Model file for the job. Use its own axes, mm. Face numbers are marked on the shaded views. A direction names the side the tool comes from. Give positions to 0.01 mm unless a question says otherwise; leave off trailing zeros. Write each loop counter-clockwise with the first axis right and the second up, starting at its lowest first coordinate (ties: lowest second). Pieces come first, ordered by that corner, then holes. Notation, with made-up numbers: (-14, -16) - (19, -16) arc R24 ccw to (19, 0) - close; hole circle Ø10 at (77.25, -16.5). An arc over 180 degrees is marked (long way). One line per item, written item: value. Start each with the question number.
(1) Probe L1, parallel to X at y = 6.5, z = -23; L2, parallel to Z at x = 8, y = 15.5; L3, parallel to X at y = 6.5, z = -20.5. List the from-to ranges inside material, lowest first.
(2) Cut at D-D, the plane x = 8. List the corners of the cut face in (y, z).
(3) Drop flat-ended pins along their axis: P1, Ø9.5, axis at x = 5, y = -4.5, coming from the -Z side; P2, Ø4, axis at x = 25.5, y = 2.5, coming from the +Z side; P3, Ø9.5, axis at y = -5.5, z = -15, coming from the +X side; P4, Ø4, axis at x = 26, z = -18.5, coming from the +Y side. Give the stop position or say it passes through.
(4) 3-axis set-ups, long thin cutter, end or side, ignore diameter. For the marked faces 4, 5 and 6: which of +Z, -Z, +X, -X, +Y, -Y reach the whole face in a straight line?
(5) Cut at C-C, the plane y = -5. List the corners of the cut face in (x, z), and give its area (3 significant figures).
(6) Cut at A-A, the plane y = 2. List the corners of the cut face in (x, z), and give its area (3 significant figures).
(7) Mould opens along X. For the marked faces 1, 2 and 3 say: pulls with the +X half, pulls with the -X half, needs draft (parallel to the pull), parting line crosses it, or undercut.
(8) Cut at B-B, the plane x = 3. List the corners of the cut face in (y, z), and give its area (3 significant figures).
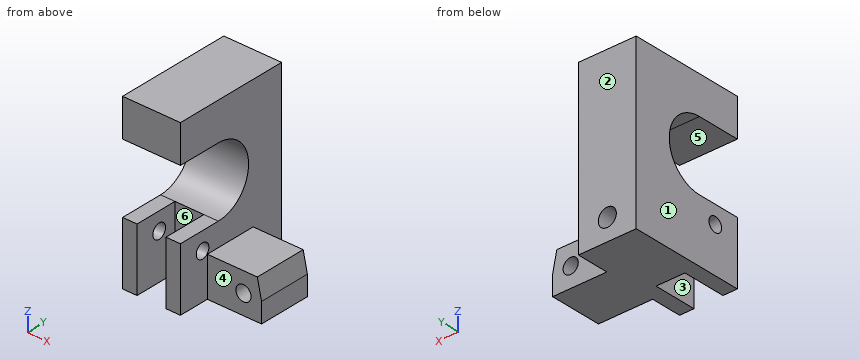
from build123d import *

# Parameters (mm, degrees)
F1_DEPTH  = 16
F2_W      = 14.5
F2_H      = 11
F3_DEPTH  = 15
F5_DEPTH  = 23.501
F7_D      = 4.2
F8_W      = 8
F8_H      = 12
F9_DEPTH  = 17.451
F10_R     = 2
F11_DEPTH = 31.001
F14_D     = 5


with BuildPart() as f1:
    # F0 (on Right) → F1 (new body)
    with BuildSketch(Plane.YZ):
        with BuildLine():
            ThreePointArc((0, 9.55), (9.55, 0), (0, -9.55))
            Line((0, -9.55), (-12, -9.55))
            Line((-12, -9.55), (-12, -27))
            Line((-12, -27), (20, -27))
            Line((20, -27), (20, 20))
            Line((20, 20), (-12, 20))
            Line((-12, 20), (-12, 9.55))
            Line((-12, 9.55), (0, 9.55))
        make_face()
    extrude(amount=F1_DEPTH)

    # F2 (on face) → F3 (join)
    with BuildSketch(Plane.YZ.offset(16)):
        with Locations((3.75, -21.5)):
            Rectangle(F2_W, F2_H)
    extrude(amount=F3_DEPTH)

    # F4 (on face) → F5 (cut, through all)
    with BuildSketch(Plane.XZ.offset(3.5)):
        Polygon((29.8309389108, -16), (31, -21.5), (31, -16), align=None)
    extrude(amount=-F5_DEPTH, mode=Mode.SUBTRACT)

    # F7 (through all)
    with Locations(Plane(origin=(0, 11, 0), x_dir=(-1, 0, 0), z_dir=(0, 1, 0))):
        with Locations((-26, -21.5)):
            Hole(F7_D / 2)

    # F8 (on face) → F9 (cut, through all)
    with BuildSketch(Plane.XY.offset(-9.55)):
        with Locations((8, -6)):
            Rectangle(F8_W, F8_H)
    extrude(amount=-F9_DEPTH, mode=Mode.SUBTRACT)

    # F10 (on face) → F11 (cut, through all)
    with BuildSketch(Plane(origin=(0, 0, 0), x_dir=(0, -1, 0), z_dir=(-1, 0, 0))):
        with Locations((5, -14.5)):
            Circle(F10_R)
    extrude(amount=-F11_DEPTH, mode=Mode.SUBTRACT)

    # F14 (through all)
    with Locations(Plane(origin=(0, 20, 0), x_dir=(-1, 0, 0), z_dir=(0, 1, 0))):
        with Locations((-8, -21)):
            Hole(F14_D / 2)


solid = f1.part
Answers follow:
1. L1: x = 0 to 6.5, 9.5 to 24.53, 27.47 to 31
1. L2: z = -27 to -23.5, -18.5 to 20
1. L3: x = 0 to 5.55, 10.45 to 24.15, 27.85 to 30.79
2. outline: (-12, 9.55) - (0, 9.55) arc R9.55 cw to (0, -9.55) - (0, -18.5) - (20, -18.5) - (20, 20) - (-12, 20) - close; (0, -27) - (20, -27) - (20, -23.5) - (0, -23.5) - close
3. P1: stops at z = -27
3. P2: stops at z = -16
3. P3: stops at x = 30.53
3. P4: stops at y = 11
4. face 4: +Z, -Z, +X, -Y
4. face 5: +X, -X, -Y
4. face 6: -Z, -Y
5. outline: (0, -27) - (4, -27) - (4, -16.5) - (0, -16.5) - close; (0, -12.5) - (4, -12.5) - (4, -9.55) - (0, -9.55) - close; (0, 9.55) - (16, 9.55) - (16, 20) - (0, 20) - close; (12, -27) - (16, -27) - (16, -16.5) - (12, -16.5) - close; (12, -12.5) - (16, -12.5) - (16, -9.55) - (12, -9.55) - close
5. area: 275 mm²
6. outline: (0, -27) - (31, -27) - (31, -21.5) - (29.83, -16) - (16, -16) - (16, -9.34) - (0, -9.34) - close; (0, 9.34) - (16, 9.34) - (16, 20) - (0, 20) - close; hole circle Ø5 at (8, -21); hole circle Ø4.2 at (26, -21.5)
6. area: 581 mm²
7. face 1: pulls with the -X half
7. face 2: needs draft
7. face 3: undercut
8. outline: (-12, -27) - (20, -27) - (20, 20) - (-12, 20) - (-12, 9.55) - (0, 9.55) arc R9.55 cw to (0, -9.55) - (-12, -9.55) - close; hole circle Ø4 at (-5, -14.5)
8. area: 1,120 mm²
